Here's how the part is built. I have some questions about the finished solid (model axes, mm). Face numbers are marked on the shaded views. Coordinates: 2 decimals unless noted, no trailing zeros. Loops run counter-clockwise (first coordinate to the right, second up) from the corner with the lowest first, then second, coordinate; pieces in that order, holes last. Notation, with made-up numbers: (-32.75, 20.5) -> (-10.75, 20.5) arc R18 ccw to (-10.75, 51.5) -> close; hole circle Ø8 at (63, 5.5). An arc over 180 degrees is marked (long way). Use CSV: the item, a comma, the result in double quotes. Start each with the question number.
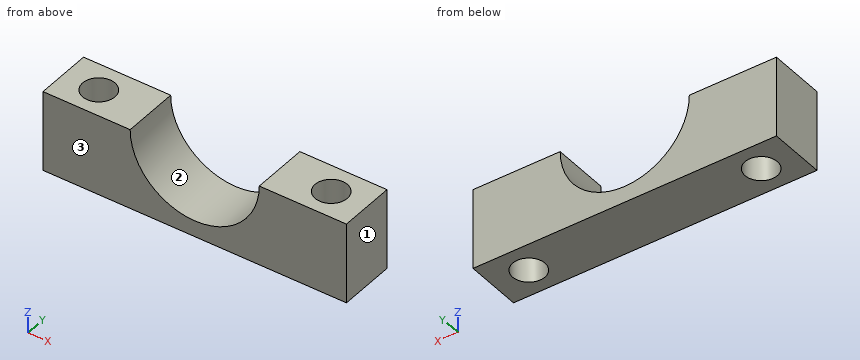
from build123d import *

# Parameters (mm, degrees)
BOSS_EXTRUDE1_DEPTH = 5.5626
SKETCH2_R           = 3.175
CUT_EXTRUDE1_DEPTH  = 16.875


with BuildPart() as part:
    # Sketch1 → Boss-Extrude1 (new body, symmetric)
    with BuildSketch(Plane(origin=(0, 0, 0), x_dir=(1, 0, 0), z_dir=(0, 1, 0))):
        with BuildLine():
            Line((-12.7, 0), (-29.845, 0))
            Line((-29.845, 0), (-29.845, 15.875))
            Line((-29.845, 15.875), (29.845, 15.875))
            Line((29.845, 15.875), (29.845, 0))
            Line((29.845, 0), (12.7, 0))
            ThreePointArc((12.7, 0), (0, 12.7), (-12.7, 0))
        make_face()
    extrude(amount=BOSS_EXTRUDE1_DEPTH, both=True)

    # Sketch2 → Cut-Extrude1 (cut, through all)
    with BuildSketch(Plane.XY):
        with Locations((-22.86, 0)):
            Circle(SKETCH2_R)
        with Locations((22.86, 0)):
            Circle(SKETCH2_R)
    extrude(amount=-CUT_EXTRUDE1_DEPTH, mode=Mode.SUBTRACT)


solid = part.part
1) Please list where these lines run through material, in increasing order: L1, parallel to X at y = 2.25, z = -1.25 (3 decimals); L2, parallel to X at y = 3.5, z = -10 (3 decimals); L3, parallel to X at y = -1.5, z = -14.25 (3 decimals). Write a range as [from, to].
2) Thinking about a two-plate mould opening in X: for the marked faces 1, 2 and 3, which applies, pulls with the +X half, pulls with the -X half, needs draft (parallel to the pull), parting line crosses it, or undercut?
3) I want a section at A-A, the plane y = 0. Please give me the cut outline in (x, z) (3 decimals).
4) I want a section at C-C, the plane z = -4. Please give me the cut outline in (x, y) (3 decimals).
5) I want a section at B-B, the plane x = 22.86. Please give me the cut outline in (y, z) (3 decimals).
6) I want a section at D-D, the plane z = -14. Please give me the cut outline in (x, y) (3 decimals).
7) For P1, Ø4, axis at x = -22.86, y = 0, coming from the -Z side, with a flat end and sliding along its axis, tell me the tip position at first contact or that it passes through.
Return value:
1,L1,"x = [-29.845, -25.1], [-20.62, -12.638], [12.638, 20.62], [25.1, 29.845]"
1,L2,"x = [-29.845, -7.829], [7.829, 29.845]"
1,L3,"x = [-29.845, -25.658], [-20.062, 20.062], [25.658, 29.845]"
2,face 1,"pulls with the +X half"
2,face 2,"undercut"
2,face 3,"needs draft"
3,outline,"(-29.845, -15.875) -> (-26.035, -15.875) -> (-26.035, 0) -> (-29.845, 0) -> close; (-19.685, -15.875) -> (19.685, -15.875) -> (19.685, 0) -> (12.7, 0) arc R12.7 cw to (-12.7, 0) -> (-19.685, 0) -> close; (26.035, -15.875) -> (29.845, -15.875) -> (29.845, 0) -> (26.035, 0) -> close"
4,outline,"(-29.845, -5.563) -> (-12.054, -5.563) -> (-12.054, 5.563) -> (-29.845, 5.563) -> close; (12.054, -5.563) -> (29.845, -5.563) -> (29.845, 5.563) -> (12.054, 5.563) -> close; hole circle Ø6.35 at (-22.86, 0); hole circle Ø6.35 at (22.86, 0)"
5,outline,"(-5.563, -15.875) -> (-3.175, -15.875) -> (-3.175, 0) -> (-5.563, 0) -> close; (3.175, -15.875) -> (5.563, -15.875) -> (5.563, 0) -> (3.175, 0) -> close"
6,outline,"(-29.845, -5.563) -> (29.845, -5.563) -> (29.845, 5.563) -> (-29.845, 5.563) -> close; hole circle Ø6.35 at (-22.86, 0); hole circle Ø6.35 at (22.86, 0)"
7,P1,"passes through"
